Answer from the drawing. Dimensions are ordinates in mm from the lowest x, y and z of the part. A direction names the side the tool comes from. Give positions to 0.01 mm unless a question says otherwise; leave off trailing zeros. Loops run counter-clockwise (first coordinate to the right, second up) from the corner with the lowest first, then second, coordinate; pieces in that order, holes last.
Item 1: Section A-A, the plane z = 5 is taken. Give the vertices of the cut face in (x, y), and give its area (3 significant figures).
Item 2: A tool of negligible diameter and unlimited length cuts with its end or side. For the marked faces 1, 2 and 3, from which of +Z, -Z, +X, -X, +Y, -Y can it reach the whole face along a straight path? Write none if from no direction.
Item 3: Section D-D, the plane x = 41 is taken. Give the vertices of the cut face in (y, z), and give its area (3 significant figures).
Item 4: Each of these flat-tipped pins is pushed along its axis until it touches: pin 1 Ø3 at (x, z) = (4.5, 5) entering from +Y; pin 2 Ø2 at (x, y) = (35.5, 4) entering from -Z; pin 3 Ø1 at (x, y) = (18, 3.5) entering from +Z; pin 4 Ø3 at (x, y) = (29.5, 7) entering from -Z. Where does it stop, or does it pass through?
Item 5: Section C-C, the plane y = 2.75 is taken. Give the vertices of the cut face in (x, z), and give its area (3 significant figures).
Item 6: Consider line 1 along X through (y, z) = (1.65, 5); line 2 along X through (y, z) = (3.75, 6.5); line 3 along Y through (x, z) = (46.5, 2.25). Determine where each line is inside the solid, lowest interval first.
Item 7: Section B-B, the plane x = 4.5 is taken. Give the vertices of the cut face in (y, z).
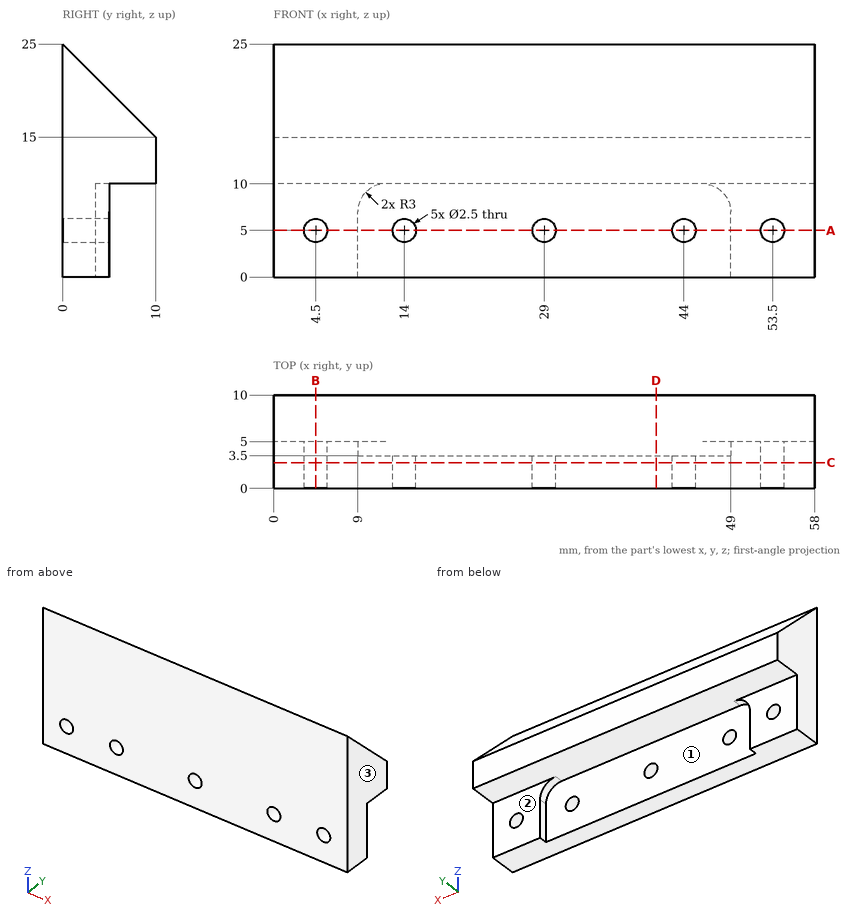
Worked answers:
1. outline: (0, 0) - (3.25, 0) - (3.25, 5) - (0, 5) - close; (5.75, 0) - (12.75, 0) - (12.75, 3.5) - (9, 3.5) - (9, 5) - (5.75, 5) - close; (15.25, 0) - (27.75, 0) - (27.75, 3.5) - (15.25, 3.5) - close; (30.25, 0) - (42.75, 0) - (42.75, 3.5) - (30.25, 3.5) - close; (45.25, 0) - (52.25, 0) - (52.25, 5) - (49, 5) - (49, 3.5) - (45.25, 3.5) - close; (54.75, 0) - (58, 0) - (58, 5) - (54.75, 5) - close
1. area: 179 mm2
2. face 1: -Z, +Y
2. face 2: -Z, +X, -X, +Y
2. face 3: +Z, -Z, +X, +Y, -Y
3. outline: (0, 0) - (3.5, 0) - (3.5, 10) - (10, 10) - (10, 15) - (0, 25) - close
3. area: 135 mm2
4. pin 1: stops at y = 5
4. pin 2: stops at z = 0
4. pin 3: stops at z = 22
4. pin 4: stops at z = 10
5. outline: (0, 0) - (58, 0) - (58, 22.25) - (0, 22.25) - close; hole circle Ø2.5 at (4.5, 5); hole circle Ø2.5 at (14, 5); hole circle Ø2.5 at (29, 5); hole circle Ø2.5 at (44, 5); hole circle Ø2.5 at (53.5, 5)
5. area: 1,270 mm2
6. line 1: x = 0 to 3.25, 5.75 to 12.75, 15.25 to 27.75, 30.25 to 42.75, 45.25 to 52.25, 54.75 to 58
6. line 2: x = 0 to 9, 49 to 58
6. line 3: y = 0 to 3.5
7. outline: (0, 0) - (5, 0) - (5, 3.75) - (0, 3.75) - close; (0, 6.25) - (5, 6.25) - (5, 10) - (10, 10) - (10, 15) - (0, 25) - close
